Read the model definition and answer for the solid it produces. Units are mm, in the model's axes. Face numbers are marked on the shaded views. A direction names the side the tool comes from. Coordinates: 2 decimals unless noted, no trailing zeros. Loops run counter-clockwise (first coordinate to the right, second up) from the corner with the lowest first, then second, coordinate; pieces in that order, holes last. Notation, with made-up numbers: (1, -27.75) - (24, -27.75) arc R23 ccw to (24, -17.75) - close; hole circle Ø8 at (41.25, 60). An arc over 180 degrees is marked (long way). One line per item, written item: value. Start each with the question number.
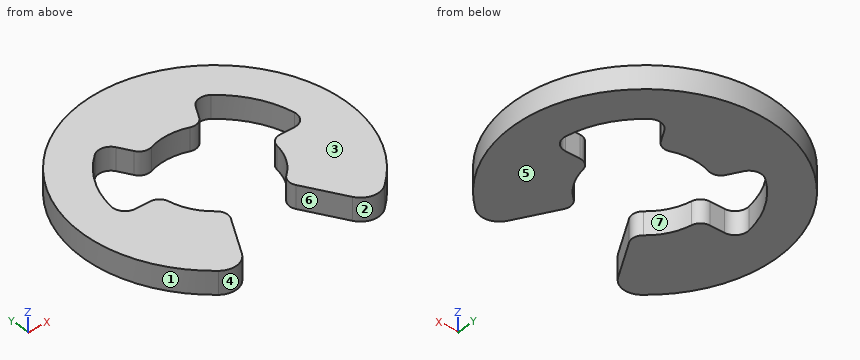
from build123d import *

# Parameters (mm, degrees)
BOSS_EXTRUDE1_DEPTH      = 0.55245
BOSS_EXTRUDE1_DEPTH_BACK = 0.55245


with BuildPart() as part:
    # Sketch1 → Boss-Extrude1 (new body, two sides)
    with BuildSketch(Plane.XY) as boss_extrude1_sk:
        with BuildLine():
            Line((-2.686207619, -4.652648077), (-1.581575189, -2.739368583))
            ThreePointArc((-1.581575189, -2.739368583), (-1.518398027, -2.377324451), (-1.703844152, -2.060027992))
            ThreePointArc((-1.703844152, -2.060027992), (-2.315189002, -1.336675019), (-2.635958642, -0.445558366))
            ThreePointArc((-2.635958642, -0.445558366), (-2.818022364, -0.126309053), (-3.163150378, 0))
            Line((-3.163150378, 0), (-3.863567646, 0))
            ThreePointArc((-3.863567646, 0), (-4.32048273, 0.210277956), (-4.457962671, 0.694103832))
            ThreePointArc((-4.457962671, 0.694103832), (-3.907225167, 2.255837494), (-2.830092898, 3.513656997))
            ThreePointArc((-2.830092898, 3.513656997), (-2.342347424, 3.636508824), (-1.931783823, 3.345947731))
            Line((-1.931783823, 3.345947731), (-1.581575189, 2.739368583))
            ThreePointArc((-1.581575189, 2.739368583), (-1.299624349, 2.503633488), (-0.932114488, 2.505586319))
            ThreePointArc((-0.932114488, 2.505586319), (-1.7e-08, 2.67335), (0.932114457, 2.505586331))
            ThreePointArc((0.932114457, 2.505586331), (1.299624333, 2.503633482), (1.581575189, 2.739368583))
            Line((1.581575189, 2.739368583), (1.931783823, 3.345947731))
            ThreePointArc((1.931783823, 3.345947731), (2.342347445, 3.636508828), (2.830092931, 3.51365697))
            ThreePointArc((2.830092931, 3.51365697), (3.907225174, 2.255837482), (4.457962669, 0.694103846))
            ThreePointArc((4.457962669, 0.694103846), (4.320482735, 0.210277961), (3.863567646, 0))
            Line((3.863567646, 0), (3.163150378, 0))
            ThreePointArc((3.163150378, 0), (2.818022373, -0.126309046), (2.635958646, -0.445558343))
            ThreePointArc((2.635958646, -0.445558343), (2.315189019, -1.33667499), (1.703844185, -2.060027965))
            ThreePointArc((1.703844185, -2.060027965), (1.518398031, -2.377324429), (1.581575189, -2.739368583))
            Line((1.581575189, -2.739368583), (2.686207619, -4.652648077))
            ThreePointArc((2.686207619, -4.652648077), (3.307353322, -5.089462883), (4.042024336, -4.897401277))
            ThreePointArc((4.042024336, -4.897401277), (-2e-08, 6.35), (-4.042024306, -4.897401302))
            ThreePointArc((-4.042024306, -4.897401302), (-3.307353303, -5.08946288), (-2.686207619, -4.652648077))
        make_face()
    extrude(amount=BOSS_EXTRUDE1_DEPTH)
    extrude(boss_extrude1_sk.sketch, amount=-BOSS_EXTRUDE1_DEPTH_BACK)


solid = part.part
1) Straight lines are drawn through the part: L1, parallel to X at y = 3, z = 0.2; L2, parallel to X at y = -3.5, z = -0.2; L3, parallel to X at y = 1.75, z = 0.1. For each, find the intervals that lie inside material, in ascending order.
2) Determine the mould class of the marked faces 1, 2, 3 and 4 for opening direction X: released by +X, released by -X, zero draft, split by the parting line, or undercut.
3) For the marked faces 5, 6 and 7, determine the directions among +Z, -Z, +X, -X, +Y, -Y from which every point of the face is accessible in a straight line to the end or side of a thin tool.
4) A flat-ended cylindrical pin translates along its axis: P1, Ø0.6, axis at x = -3.5, z = 0, coming from the +Y side. Find the tip coordinate at first contact, or state that the pin passes through.
5) Section A-A, the plane y = -2.25 is taken. Determine the outline of the cut face in (x, z).
6) Section C-C, the plane x = 0 is taken. Determine the outline of the cut face in (y, z), and give its area (3 significant figures).
7) Section D-D, the plane x = -4.75 is taken. Determine the outline of the cut face in (y, z).
8) Section B-B, the plane z = -0.4 is taken. Determine the outline of the cut face in (x, y).
Answer below:
1. L1: -5.6 to -3.37, -1.73 to 1.73, 3.37 to 5.6
1. L2: -5.3 to -2.02, 2.02 to 5.3
1. L3: -6.1 to -4.16, 4.16 to 6.1
2. face 1: split by the parting line
2. face 2: undercut
2. face 3: zero draft
2. face 4: undercut
3. face 5: -Z, +X, -X, +Y, -Y
3. face 6: +Z, -Z, -Y
3. face 7: +Z, -Z
4. P1: y = 5.48
5. outline: (-5.94, -0.55) - (-1.56, -0.55) - (-1.56, 0.55) - (-5.94, 0.55) - close; (1.56, -0.55) - (5.94, -0.55) - (5.94, 0.55) - (1.56, 0.55) - close
6. outline: (2.67, -0.55) - (6.35, -0.55) - (6.35, 0.55) - (2.67, 0.55) - close
6. area: 4.06 mm2
7. outline: (-4.21, -0.55) - (4.21, -0.55) - (4.21, 0.55) - (-4.21, 0.55) - close
8. outline: (-4.46, 0.69) arc R4.51 cw to (-2.83, 3.51) arc R0.6 cw to (-1.93, 3.35) - (-1.58, 2.74) arc R0.53 ccw to (-0.93, 2.51) arc R2.67 cw to (0.93, 2.51) arc R0.53 ccw to (1.58, 2.74) - (1.93, 3.35) arc R0.6 cw to (2.83, 3.51) arc R4.51 cw to (4.46, 0.69) arc R0.6 cw to (3.86, 0) - (3.16, 0) arc R0.53 ccw to (2.64, -0.45) arc R2.67 cw to (1.7, -2.06) arc R0.53 ccw to (1.58, -2.74) - (2.69, -4.65) arc R0.9 ccw to (4.04, -4.9) arc R6.35 ccw (long way) to (-4.04, -4.9) arc R0.9 ccw to (-2.69, -4.65) - (-1.58, -2.74) arc R0.53 ccw to (-1.7, -2.06) arc R2.67 cw to (-2.64, -0.45) arc R0.53 ccw to (-3.16, 0) - (-3.86, 0) arc R0.6 cw to start
